Verification items for this drawing (mm, ordinates from the low corner). Coordinates: 2 decimals unless noted, no trailing zeros. Write each loop counter-clockwise with the first axis right and the second up, starting at its lowest first coordinate (ties: lowest second). Pieces come first, ordered by that corner, then holes.
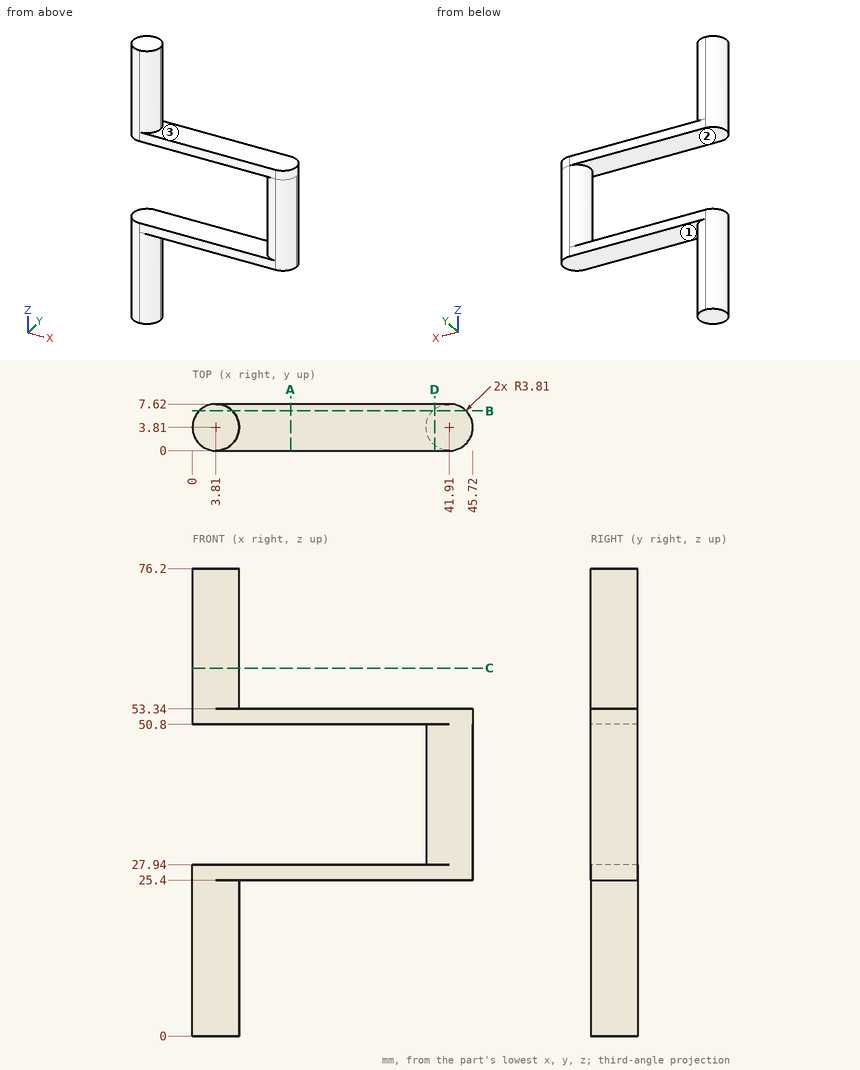
1. Sectioned sample at D-D, the plane x = 39.5. Record the boundary of the cut face in (y, z).
Computed values:
outline: (0, 25.4) - (7.62, 25.4) - (7.62, 27.94) - (6.76, 27.94) - (6.76, 50.8) - (7.62, 50.8) - (7.62, 53.34) - (0, 53.34) - (0, 50.8) - (0.86, 50.8) - (0.86, 27.94) - (0, 27.94) - close
2. Sectioned sample at A-A, the plane x = 16. Record the boundary of the cut face in (y, z), and give its area (3 significant figures).
Computed values:
outline: (0, 25.4) - (7.62, 25.4) - (7.62, 27.94) - (0, 27.94) - close; (0, 50.8) - (7.62, 50.8) - (7.62, 53.34) - (0, 53.34) - close
area: 38.7 mm2
3. Draft check along Z on the marked faces 1, 2 and 3. Enter one of: released by +Z, released by -Z, zero draft, split by the parting line, or undercut.
Computed values:
face 1: released by -Z
face 2: undercut
face 3: released by +Z
4. Gauge pin test, flat ends, axial feed: pin 1 Ø4 at (x, y) = (37.5, 6) entering from -Z; pin 2 Ø2.5 at (x, y) = (25.5, 5) entering from +Z; pin 3 Ø1 at (y, z) = (6.5, 10) entering from -X. Record the tip position at first contact, or that the pin passes through.
Computed values:
pin 1: stops at z = 25.4
pin 2: stops at z = 53.34
pin 3: stops at x = 0.69
5. Thickness scan on line 1 along Z through (x, y) = (28.5, 7); line 2 along Z through (x, y) = (3.5, 6.75); line 3 along X through (y, z) = (4, 25). Record the ranges inside material, lowest first.
Computed values:
line 1: z = 25.4 to 27.94, 50.8 to 53.34
line 2: z = 0 to 27.94, 50.8 to 76.2
line 3: x = 0 to 7.62
6. Sectioned sample at B-B, the plane y = 6.5. Record the boundary of the cut face in (x, z).
Computed values:
outline: (1.11, 0) - (6.51, 0) - (6.51, 25.4) - (44.61, 25.4) - (44.61, 53.34) - (6.51, 53.34) - (6.51, 76.2) - (1.11, 76.2) - (1.11, 50.8) - (39.21, 50.8) - (39.21, 27.94) - (1.11, 27.94) - close
7. Sectioned sample at C-C, the plane z = 60. Record the boundary of the cut face in (x, y).
Computed values:
outline: (3.81, 0) arc R3.81 ccw to (7.62, 3.81) arc R3.81 ccw (long way) to start
